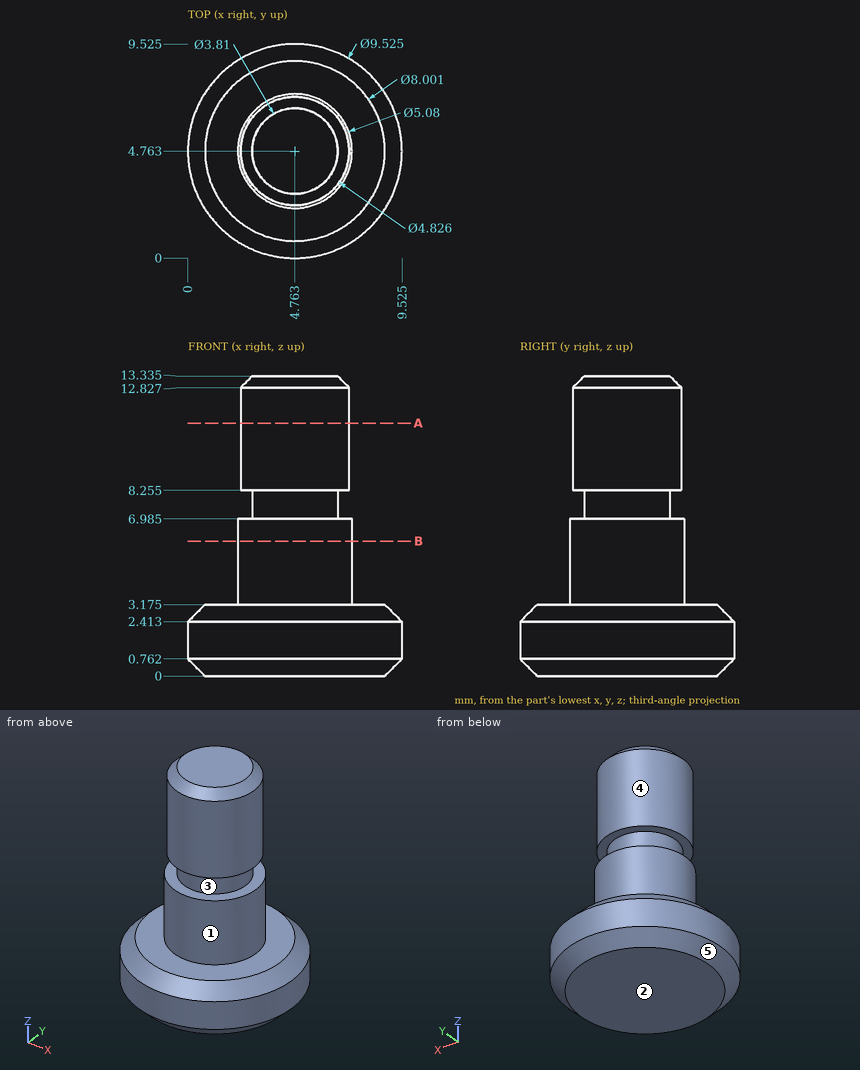
Part print with two shaded views. Sizes in mm from the minimum x, y, z corner. A direction names the side the tool comes from. Round coordinates to 2 decimals unless told otherwise and drop trailing zeros. Order: outer loops, then holes, each group sorted by start corner. A loop starts at its lowest first (then second) coordinate and runs counter-clockwise, first axis right, second up. Notation, with made-up numbers: M -23.5,35 L -5.5,35 A21 cw -5.5,52 Z; hole C -19,47.5 d4. An arc over 180 degrees is marked long. Use CSV: the item, a comma, the result in double quotes. Start each with the question number.
(1) Drill centre lines: probe 1 along Z at (x, y) = (3.25, 1.75) (1 decimal); probe 2 along Z at (x, y) = (7.25, 5) (1 decimal); probe 3 along Z at (x, y) = (2.75, 3.5) (1 decimal). Where is each one in solid material? Low to high.
(2) Cut at A-A on z = 11.25. List the corners of the cut face in (x, y) (1 decimal), then the cut area to 3 significant figures.
(3) Flat gauge pins, fed straight in: P1, Ø4, axis at x = 8, y = 1.5, coming from the -Z side; P2, Ø4, axis at x = 7.5, z = 1.5, coming from the +Y side; P3, Ø3, axis at y = 7, z = 5.5, coming from the -X side; P4, Ø3, axis at y = 5.5, z = 6, coming from the +X side. Where does each tip first touch, or does it go through?
(4) Mould opens along Z. For the marked faces 3, 4 and 5 say: +Z half, -Z half, draft (parallel to the pull), parting line (faces both ways), or undercut.
(5) Tool access for the marked faces 1 and 2: list every direction of +Z, -Z, +X, -X, +Y, -Y with a clear straight run to the whole face (end or side of a thin tool).
(6) Cut at B-B on z = 6. List the corners of the cut face in (x, y).
Findings:
1,probe 1,"z = 0 to 3.2"
1,probe 2,"z = 0 to 7"
1,probe 3,"z = 0 to 7, 8.3 to 12.9"
2,outline,"C 4.8,4.8 d4.8"
2,area,"18.3 mm^2"
3,P1,"stops at z = 0"
3,P2,"stops at y = 9.47"
3,P3,"stops at x = 2.33"
3,P4,"stops at x = 7.3"
4,face 3,"undercut"
4,face 4,"draft"
4,face 5,"-Z half"
5,face 1,"+Z"
5,face 2,"-Z, +X, -X, +Y, -Y"
6,outline,"C 4.76,4.76 d5.08"
